Work out the finished part from the listing and answer in its coordinate system (mm). Face numbers are marked on the shaded views. A direction names the side the tool comes from. Round coordinates to 2 decimals unless told otherwise and drop trailing zeros. Loops run counter-clockwise (first coordinate to the right, second up) from the corner with the lowest first, then second, coordinate; pieces in that order, holes last.
```python
from build123d import *

# Parameters (mm, degrees)
F1_DEPTH  = 30.48
F2_R      = 1.42875
F3_DEPTH  = 67.945
F4_R      = 5.08
F5_R      = 5.08
F6_R      = 5.08
F7_SIZE   = 0.98552
F8_R      = 2.50825
F9_DEPTH  = 18.161
F10_W     = 3.302
F10_H     = 17.272
F11_DEPTH = 16.3322
F12_R     = 5.08
F13_R     = 7.62
F14_R     = 7.62
F16_DEPTH = 25.4


# Not quite as in the source:
# - a feature names something its author has since deleted; it is built from what else it names


with BuildPart() as f1:
    # F0 (on Front) → F1 (new body)
    with BuildSketch(Plane.XZ):
        Polygon((-20.2290668074, 29.0888086691), (-25.3090668074, 29.0888086691), (-25.3090668074, -15.3611913309), (23.3149106546, -15.3611913309), (23.3149106546, 29.0888086691), (18.2349106546, 29.0888086691), (18.2349106546, -10.2811913309), (-20.2290668074, -10.2811913309), align=None)
    extrude(amount=F1_DEPTH)

    # F2 (on face) → F3 (cut)
    with BuildSketch(Plane.YZ.offset(23.3149106546)):
        with Locations((-21.17725, 9.5689086691)):
            Circle(F2_R)
        with BuildLine():
            ThreePointArc((-7.874, 9.5689086691), (-9.30275, 10.9976586691), (-10.7315, 9.5689086691))
            ThreePointArc((-10.7315, 9.5689086691), (-9.30275, 8.1401586691), (-7.874, 9.5689086691))
        make_face()
    extrude(amount=-F3_DEPTH, mode=Mode.SUBTRACT)

    # F4
    f4_edges = [f1.edges().sort_by_distance(p)[0] for p in [
        (20.774911, 0, 29.088809),
        (20.774911, -30.48, 29.088809),
    ]]
    fillet(f4_edges, radius=F4_R)

    # F5
    f5_edges = [f1.edges().sort_by_distance(p)[0] for p in [
        (23.314911, -15.24, -15.361191),
        (18.234911, -15.24, -10.281191),
    ]]
    fillet(f5_edges, radius=F5_R)

    # F6
    f6_edges = [f1.edges().sort_by_distance(p)[0] for p in [
        (-20.229067, -15.24, -10.281191),
        (-25.309067, -15.24, -15.361191),
    ]]
    fillet(f6_edges, radius=F6_R)

    # F7
    f7_edges = [f1.edges().sort_by_distance(p)[0] for p in [
        (18.234911, -7.874, 9.568909),
        (18.234911, -22.606, 9.568909),
    ]]
    chamfer(f7_edges, length=F7_SIZE)

    # F8 (on face) → F9 (cut)
    with BuildSketch(Plane(origin=(-25.3090668074, 0, 0), x_dir=(0, -1, 0), z_dir=(-1, 0, 0))):
        with Locations((21.17725, 9.5689086691)):
            Circle(F8_R)
        with Locations((9.30275, 9.5689086691)):
            Circle(F8_R)
    extrude(amount=-F9_DEPTH, mode=Mode.SUBTRACT)

    # F10 (on face) → F11 (join)
    with BuildSketch(Plane.YZ.offset(-20.2290668074)):
        with Locations((-11.938, 20.4528086691)):
            Rectangle(F10_W, F10_H)
        with Locations((-18.542, 20.4528086691)):
            Rectangle(F10_W, F10_H)
    extrude(amount=F11_DEPTH)

    # F12
    f12_edges = [f1.edges().sort_by_distance(p)[0] for p in [
        (-22.769067, 0, 29.088809),
        (-22.769067, -30.48, 29.088809),
    ]]
    fillet(f12_edges, radius=F12_R)

    # F13
    f13_edges = [f1.edges().sort_by_distance(p)[0] for p in [
        (-3.896867, -11.938, 29.088809),
        (-3.896867, -11.938, 11.816809),
    ]]
    fillet(f13_edges, radius=F13_R)

    # F14
    f14_edges = [f1.edges().sort_by_distance(p)[0] for p in [
        (-3.896867, -18.542, 29.088809),
        (-3.896867, -18.542, 11.816809),
    ]]
    fillet(f14_edges, radius=F14_R)

    # F15 (on face) → F16 (cut)
    with BuildSketch(Plane(origin=(0, -10.287, 0), x_dir=(-1, 0, 0), z_dir=(0, 1, 0))):
        with BuildLine():
            ThreePointArc((8.8498668074, 20.4528086691), (11.4089168074, 17.8937586691), (13.9679668074, 20.4528086691))
            ThreePointArc((13.9679668074, 20.4528086691), (11.4089168074, 23.0118586691), (8.8498668074, 20.4528086691))
        make_face()
    extrude(amount=-F16_DEPTH, mode=Mode.SUBTRACT)


solid = f1.part
```
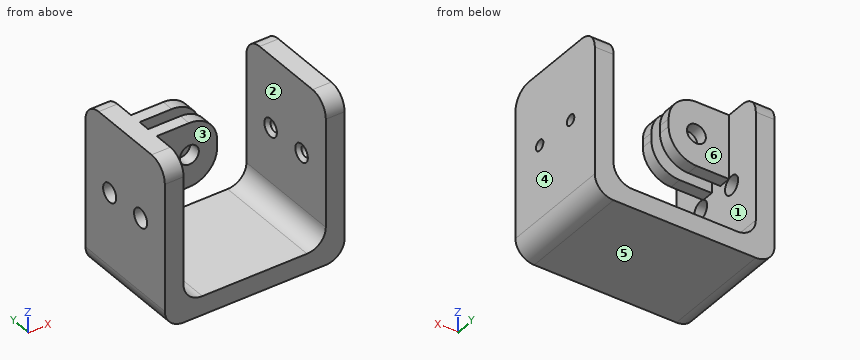
1. Which of the six approach directions +Z, -Z, +X, -X, +Y, -Y give full straight-line access (tool end or side, diameter ignored) to the marked faces 1, 2 and 3?
Answer key:
face 1: none
face 2: +Z, +Y, -Y
face 3: +Z, -Y
2. Determine the mould class of the marked faces 4, 5 and 6 for opening direction X: +X half, -X half, draft (parallel to the pull), parting line (faces both ways), or undercut.
Answer key:
face 4: +X half
face 5: draft
face 6: undercut
3. Find section D-D (z = 18.5). Write down the section's boundary in (x, y).
Answer key:
outline: (-25.31, -30.48) - (-20.23, -30.48) - (-20.23, -20.19) - (-13.06, -20.19) - (-13.06, -16.89) - (-20.23, -16.89) - (-20.23, -13.59) - (-13.06, -13.59) - (-13.06, -10.29) - (-20.23, -10.29) - (-20.23, 0) - (-25.31, 0) - close; (-9.76, -20.19) - (-3.95, -20.19) - (-3.95, -16.89) - (-9.76, -16.89) - close; (-9.76, -13.59) - (-3.95, -13.59) - (-3.95, -10.29) - (-9.76, -10.29) - close; (18.23, -30.48) - (23.31, -30.48) - (23.31, 0) - (18.23, 0) - close
4. Given pin 1 (10 mm diameter, centred on x = 11.5, z = 4.5, fed in from +Y); pin 2 (5 mm diameter, centred on x = -10, z = 23.5, fed in from -Y); pin 3 (13 mm diameter, centred on x = -9.5, z = 18, fed in from +Y); pin 4 (3 mm diameter, centred on y = -21, z = 8.5, fed in from +X), each flat-ended and moving along its own axis, determine where each tip first touches the part or whether it passes through.
Answer key:
pin 1: passes through
pin 2: stops at y = -20.19
pin 3: stops at y = -10.29
pin 4: stops at x = 23.31
5. Consider probe 1 along Y at (x, z) = (-12.5, 24); probe 2 along Z at (x, y) = (-14, -19.5); probe 3 along X at (y, z) = (-22, -1). Determine where each line is inside the solid, lowest interval first.
Answer key:
probe 1: y = -20.19 to -16.89, -13.59 to -10.29
probe 2: z = -15.36 to -10.28, 11.82 to 29.09
probe 3: x = -25.31 to -20.23, 18.23 to 23.31
6. Find section B-B (x = -5). Write down the section's boundary in (y, z).
Answer key:
outline: (-30.48, -15.36) - (0, -15.36) - (0, -10.28) - (-30.48, -10.28) - close; (-20.19, 15.49) - (-16.89, 15.49) - (-16.89, 25.42) - (-20.19, 25.42) - close; (-13.59, 15.49) - (-10.29, 15.49) - (-10.29, 25.42) - (-13.59, 25.42) - close
7. Find section A-A (z = 3). Write down the section's boundary in (x, y), then the cut area to 3 significant figures.
Answer key:
outline: (-25.31, -30.48) - (-20.23, -30.48) - (-20.23, 0) - (-25.31, 0) - close; (18.23, -30.48) - (23.31, -30.48) - (23.31, 0) - (18.23, 0) - close
area: 310 mm2
8. Find section C-C (y = -27). Write down the section's boundary in (x, z).
Answer key:
outline: (-25.31, -10.28) arc R5.08 ccw to (-20.23, -15.36) - (18.23, -15.36) arc R5.08 ccw to (23.31, -10.28) - (23.31, 28.83) - (18.23, 28.83) - (18.23, -5.2) arc R5.08 cw to (13.15, -10.28) - (-15.15, -10.28) arc R5.08 cw to (-20.23, -5.2) - (-20.23, 28.83) - (-25.31, 28.83) - close
